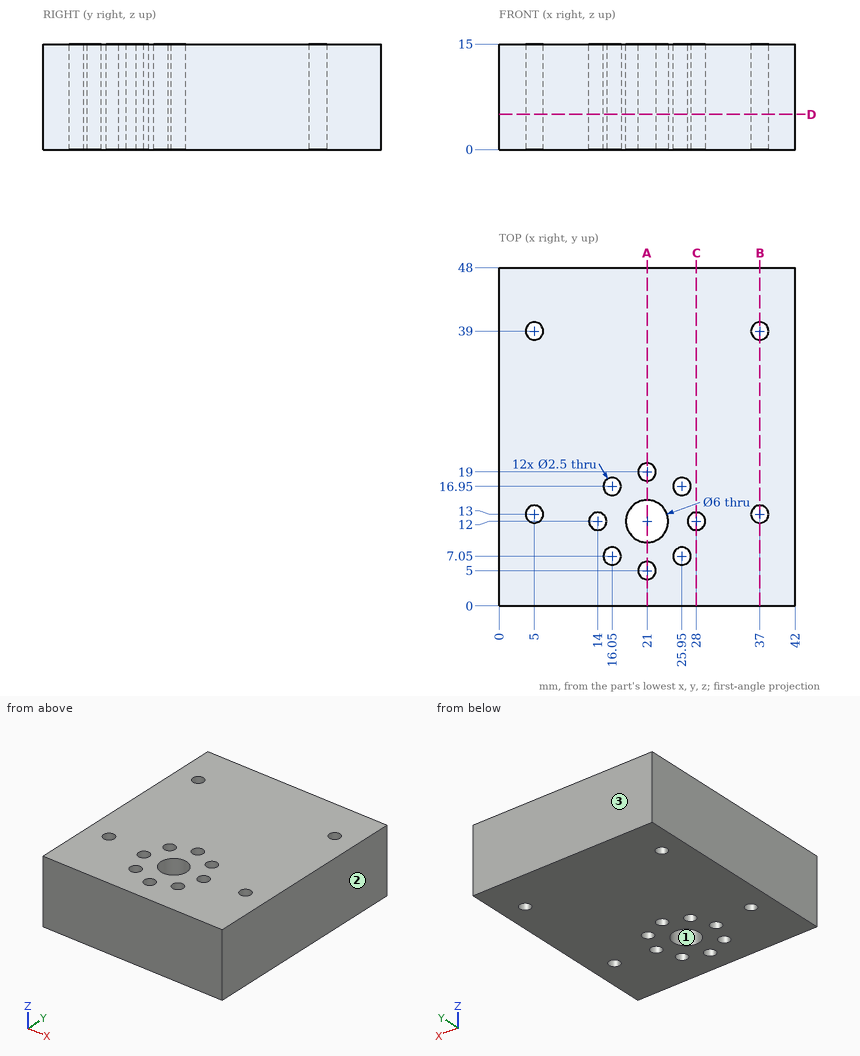
Check sheet for the drawn part. Datum: minimum x, y, z corner. Units: mm. Round coordinates to 2 decimals unless told otherwise and drop trailing zeros. Order: outer loops, then holes, each group sorted by start corner. A loop starts at its lowest first (then second) coordinate and runs counter-clockwise, first axis right, second up.
1. Section check A-A on x = 21. Record the cut outline in (y, z).
Final values:
outline: (0, 0) - (3.75, 0) - (3.75, 15) - (0, 15) - close; (6.25, 0) - (9, 0) - (9, 15) - (6.25, 15) - close; (15, 0) - (17.75, 0) - (17.75, 15) - (15, 15) - close; (20.25, 0) - (48, 0) - (48, 15) - (20.25, 15) - close
2. Thickness scan on L1, parallel to X at y = 7, z = 13.5; L2, parallel to Y at x = 26, z = 8.5; L3, parallel to Y at x = 4, z = 7.5. Record the ranges inside material, lowest first.
Final values:
L1: x = 0 to 14.8, 17.3 to 24.7, 27.2 to 42
L2: y = 0 to 5.8, 8.3 to 15.7, 18.2 to 48
L3: y = 0 to 12.25, 13.75 to 38.25, 39.75 to 48
3. Release check for a two-part mould opening along Y. For the marked faces 1, 2 and 3 record: +Y half, -Y half, draft (parallel to the pull), parting line (faces both ways), or undercut.
Final values:
face 1: undercut
face 2: draft
face 3: +Y half
4. Section check C-C on x = 28. Record the cut outline in (y, z).
Final values:
outline: (0, 0) - (10.75, 0) - (10.75, 15) - (0, 15) - close; (13.25, 0) - (48, 0) - (48, 15) - (13.25, 15) - close
5. Section check B-B on x = 37. Record the cut outline in (y, z), then the cut area to 3 significant figures.
Final values:
outline: (0, 0) - (11.75, 0) - (11.75, 15) - (0, 15) - close; (14.25, 0) - (37.75, 0) - (37.75, 15) - (14.25, 15) - close; (40.25, 0) - (48, 0) - (48, 15) - (40.25, 15) - close
area: 645 mm2
6. Section check D-D on z = 5. State how many separate pieces and enclosed holes the cut face has, then the cut area to 3 significant figures.
Final values:
separate pieces: 1
enclosed holes: 13
area: 1,930 mm2
